from build123d import *

# Parameters (mm, degrees)
BASE_FLANGE1_DEPTH           = 50.8
CUT_EXTRUDE1_DEPTH           = 61.049583679
CUT_EXTRUDE1_DEPTH_BACK      = 61.049583679
SKETCH6_W                    = 22.2
SKETCH6_H                    = 40.396012785
SKETCH6_W_2                  = 19
F_7_0_7_DIAMETER_HOLE1_D     = 7
F_7_0_7_DIAMETER_HOLE1_DEPTH = 10
F_7_0_7_DIAMETER_HOLE1_TIP   = 2.103012167
CUT_EXTRUDE2_DEPTH           = 10
CHAMFER1_SIZE                = 0.5
CHAMFER2_SIZE                = 0.5
CHAMFER2_SIZE_2              = 2.83564091


# Sheet-metal steps are written as plain solids
with BuildPart() as part:
    # Sketch1 → Base-Flange1 (new, symmetric)
    with BuildSketch(Plane(origin=(0, 0, 0), x_dir=(0, 0, -1), z_dir=(1, 0, 0))):
        with BuildLine():
            Line((31.5, -5), (4.137865616, -5))
            ThreePointArc((4.137865616, -5), (2.850262482, -5.083242558), (1.584096024, -5.331584366))
            Line((1.584096024, -5.331584366), (0.651734752, -5.577853864))
            ThreePointArc((0.651734752, -5.577853864), (-0.279113067, -5.709460074), (-1.214968707, -5.620173577))
            ThreePointArc((-1.214968707, -5.620173577), (-2.620425709, 5.118190022), (5.269962049, -2.3))
            Line((5.269962049, -2.3), (2.978674202, -1.3))
            ThreePointArc((2.978674202, -1.3), (-1.481110183, 2.892890013), (-0.686721443, -3.176619848))
            ThreePointArc((-0.686721443, -3.176619848), (-0.335775578, -3.210102284), (0.013292354, -3.160749956))
            Line((0.013292354, -3.160749956), (0.945653625, -2.914480458))
            ThreePointArc((0.945653625, -2.914480458), (2.528361698, -2.604053197), (4.137865616, -2.5))
            Line((4.137865616, -2.5), (31.5, -2.5))
            Line((31.5, -2.5), (31.5, -5))
        make_face()
    extrude(amount=BASE_FLANGE1_DEPTH, both=True)

    # Sketch6 → Cut-Extrude1 (cut, two sides: drawn at the far end of the back side and taken through both)
    with BuildSketch(Plane(origin=(0, 0, 0), x_dir=(1, 0, 0), z_dir=(0, 1, 0)).offset(-CUT_EXTRUDE1_DEPTH_BACK)):
        with Locations((-39.7, -13.198006393)):
            Rectangle(SKETCH6_W, SKETCH6_H)
        with Locations((39.7, -13.198006393)):
            Rectangle(SKETCH6_W, SKETCH6_H)
        with Locations((0, -13.198006393)):
            Rectangle(SKETCH6_W_2, SKETCH6_H)
    extrude(amount=CUT_EXTRUDE1_DEPTH + CUT_EXTRUDE1_DEPTH_BACK, mode=Mode.SUBTRACT)

    # Ø7.0 (7) Diameter Hole1
    with Locations(Plane(origin=(0, -2.5, 0), x_dir=(1, 0, 0), z_dir=(0, 1, 0))):
        with Locations((37.75, 15.65), (-37.75, 15.65), (12.25, 25.65)):
            Hole(F_7_0_7_DIAMETER_HOLE1_D / 2, depth=F_7_0_7_DIAMETER_HOLE1_DEPTH)
            with Locations((0, 0, -(F_7_0_7_DIAMETER_HOLE1_DEPTH + F_7_0_7_DIAMETER_HOLE1_TIP / 2))):  # 118° drill point
                Cone(0, F_7_0_7_DIAMETER_HOLE1_D / 2, F_7_0_7_DIAMETER_HOLE1_TIP, mode=Mode.SUBTRACT)

    # Sketch9 → Cut-Extrude2 (cut)
    with BuildSketch(Plane(origin=(0, -2.5, 0), x_dir=(1, 0, 0), z_dir=(0, 1, 0))):
        with BuildLine():
            Line((-9.15, 27.15), (-9.15, 21.15))
            ThreePointArc((-9.15, 21.15), (-12.25, 18.05), (-15.35, 21.15))
            Line((-15.35, 21.15), (-15.35, 27.15))
            ThreePointArc((-15.35, 27.15), (-12.25, 30.25), (-9.15, 27.15))
        make_face()
    extrude(amount=-CUT_EXTRUDE2_DEPTH, mode=Mode.SUBTRACT)

    # Chamfer1
    chamfer1_edges = [part.edges().sort_by_distance(p)[0] for p in [
        (15.75, -2.5, -25.65),
        (-34.25, -2.5, -15.65),
        (41.25, -2.5, -15.65),
        (-12.25, -2.5, -30.25),
        (-15.35, -2.5, -24.15),
        (-12.25, -2.5, -18.05),
        (-9.15, -2.5, -24.15),
    ]]
    chamfer(chamfer1_edges, length=CHAMFER1_SIZE)

    # Chamfer2
    # the kernel refuses this chamfer: 2.83564091, 0.5 mm, written as the material it takes off along each edge
    with BuildSketch(Plane(origin=(-28.6, -2.5, -7), x_dir=(0, 0.21013876076743535, -0.9776715712462578), z_dir=(-1, 0, 0))) as chamfer2_piece_1:
        Polygon((CHAMFER2_SIZE * 0.977671571246, CHAMFER2_SIZE * 0.210138760767), (-CHAMFER2_SIZE_2 * 0.210138760753, CHAMFER2_SIZE_2 * 0.97767157118), (0, 0), align=None)
    extrude(amount=29.568522917, mode=Mode.SUBTRACT)
    with BuildSketch(Plane(origin=(-9.5, -2.5, -7), x_dir=(0, 0.21013876076743535, -0.9776715712462578), z_dir=(1, 0, 0))) as chamfer2_piece_2:
        Polygon((CHAMFER2_SIZE * 0.977671571246, -CHAMFER2_SIZE * 0.210138760767), (-CHAMFER2_SIZE_2 * 0.210138760753, -CHAMFER2_SIZE_2 * 0.97767157118), (0, 0), align=None)
    extrude(amount=19, mode=Mode.SUBTRACT)
    with BuildSketch(Plane(origin=(28.6, -2.5, -7), x_dir=(0, 0.21013876076743535, -0.9776715712462578), z_dir=(1, 0, 0))) as chamfer2_piece_3:
        Polygon((CHAMFER2_SIZE * 0.977671571246, -CHAMFER2_SIZE * 0.210138760767), (-CHAMFER2_SIZE_2 * 0.210138760753, -CHAMFER2_SIZE_2 * 0.97767157118), (0, 0), align=None)
    extrude(amount=29.568522917, mode=Mode.SUBTRACT)


solid = part.part
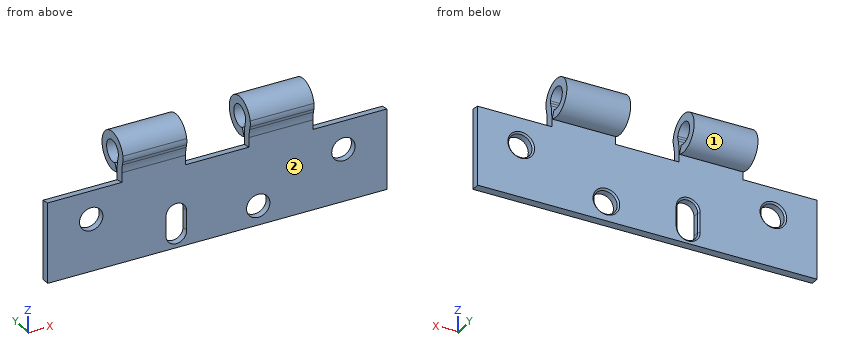
Build history of the part. All positions in model axes, mm. Face numbers are marked on the shaded views. A direction names the side the tool comes from. Coordinates: 2 decimals unless noted, no trailing zeros. Write each loop counter-clockwise with the first axis right and the second up, starting at its lowest first coordinate (ties: lowest second). Pieces come first, ordered by that corner, then holes.
(1) Cut at D-D on y = 4.5. List the corners of the cut face in (x, z), and give its area (3 significant figures).
(2) Cut at A-A on y = 0. List the corners of the cut face in (x, z), and give its area (3 significant figures).
(3) Cut at C-C on x = -12.25. List the corners of the cut face in (y, z), and give its area (3 significant figures).
(4) Cut at B-B on z = -25.65. List the corners of the cut face in (x, y), and give its area (4 significant figures).
(5) Pin check, flat tips, straight feed: pin 1 Ø6 at (x, y) = (15.5, -4) entering from +Z; pin 2 Ø22 at (x, z) = (-21, -17) entering from +Y; pin 3 Ø3 at (y, z) = (0.5, -26.5) entering from +X; pin 4 Ø11 at (x, z) = (-37.75, -15.65) entering from -Y. Stop position of each tip, or through.
(6) Drill centre lines: line 1 (X direction, y = -4.3, z = -25.65); line 2 (X direction, y = 0.25, z = -5); line 3 (Z direction, x = -14, y = 0). Where is each one in solid material? Low to high.
(7) 3-axis set-ups, long thin cutter, end or side, ignore diameter. For the marked faces 1 and 2: which of +Z, -Z, +X, -X, +Y, -Y reach the whole face in a straight line?
Working result:
1. outline: (-28.6, -3.58) - (-9.5, -3.58) - (-9.5, 3.58) - (-28.6, 3.58) - close; (9.5, -3.58) - (28.6, -3.58) - (28.6, 3.58) - (9.5, 3.58) - close
1. area: 273 mm2
2. outline: (-28.6, -5.75) - (-9.5, -5.75) - (-9.5, -3.25) - (-28.6, -3.25) - close; (-28.6, 3.25) - (-9.5, 3.25) - (-9.5, 5.75) - (-28.6, 5.75) - close; (9.5, -5.75) - (28.6, -5.75) - (28.6, -3.25) - (9.5, -3.25) - close; (9.5, 3.25) - (28.6, 3.25) - (28.6, 5.75) - (9.5, 5.75) - close
2. area: 191 mm2
3. outline: (-5.62, 1.21) arc R4 ccw to (-5.58, -0.65) - (-5.33, -1.58) arc R10 cw to (-5, -4.14) - (-5, -18.05) - (-3, -18.05) - (-2.5, -17.55) - (-2.5, -4.14) arc R12.5 ccw to (-2.91, -0.95) - (-3.16, -0.01) arc R1.5 cw to (-3.18, 0.69) arc R3.25 cw (long way) to (-1.3, -2.98) - (-2.3, -5.27) arc R5.75 ccw (long way) to start; (-5, -31.5) - (-2.5, -31.5) - (-2.5, -30.75) - (-3, -30.25) - (-5, -30.25) - close
3. area: 106 mm2
4. outline: (-50.8, -5) - (-15.35, -5) - (-15.35, -3) - (-15.85, -2.5) - (-50.8, -2.5) - close; (-9.15, -5) - (8.75, -5) - (8.75, -3) - (8.25, -2.5) - (-8.65, -2.5) - (-9.15, -3) - close; (15.75, -5) - (50.8, -5) - (50.8, -2.5) - (16.25, -2.5) - (15.75, -3) - close
4. area: 220.5 mm2
5. pin 1: stops at z = 5.66
5. pin 2: stops at y = -2.5
5. pin 3: passes through
5. pin 4: stops at y = -5
6. line 1: x = -50.8 to -15.35, -9.15 to 8.75, 15.75 to 50.8
6. line 2: x = -28.6 to -9.5, 9.5 to 28.6
6. line 3: z = -5.75 to -3.25, 3.25 to 5.75
7. face 1: +X, -X
7. face 2: -Z, +X, -X, -Y
